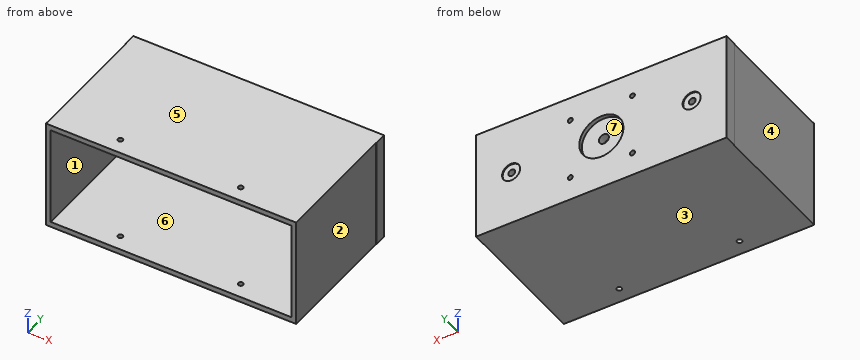
```python
from build123d import *

# Parameters (mm, degrees)
SKETCH_1_W                     = 125
SKETCH_1_H                     = 55
EXTRUDE_1_DEPTH                = 6
SKETCH_2_R                     = 11
CUT_EXTRUDE_1_DEPTH            = 2
CUT_EXTRUDE_2_REACH            = 70.4
SKETCH_3_R                     = 2.5
HOLE_WIZARD_M3_1_D             = 2.5
HOLE_WIZARD_M3_1_DEPTH         = 7.5
HOLE_WIZARD_M3_1_TIP           = 0.751075774
SKETCH_6_W                     = 124.723991502
SKETCH_6_H                     = 55
SKETCH_6_W_2                   = 120
SKETCH_6_H_2                   = 49.685135096
EXTRUDE_2_DEPTH                = 63.306419
HOLE_WIZARD_M3_2_D             = 2.5
HOLE_WIZARD_M3_2_DEPTH         = 2.657432452
HOLE_WIZARD_M3_3_D             = 2.5
HOLE_WIZARD_M3_1_2_D           = 3.4
HOLE_WIZARD_M3_1_2_DEPTH       = 5
HOLE_WIZARD_M3_1_2_CBORE_D     = 9
HOLE_WIZARD_M3_1_2_CBORE_DEPTH = 0.5
HOLE_WIZARD_M3_1_2_TIP         = 1.021463052


with BuildPart() as part:
    # 草图1 → 凸台-拉伸1 (new body)
    with BuildSketch(Plane(origin=(0, 0, 0), x_dir=(1, 0, 0), z_dir=(0, 1, 0))):
        Rectangle(SKETCH_1_W, SKETCH_1_H)
    extrude(amount=EXTRUDE_1_DEPTH)

    # 草图2 → 切除-拉伸1 (cut)
    with BuildSketch(Plane(origin=(0, 6, 0), x_dir=(1, 0, 0), z_dir=(0, 1, 0))):
        with Locations(Location((0, 0, 0), (0, 0, 270))):
            Circle(SKETCH_2_R)
    extrude(amount=-CUT_EXTRUDE_1_DEPTH, mode=Mode.SUBTRACT)

    # 草图3 → 切除-拉伸2 (cut, up to next)
    with BuildSketch(Plane(origin=(0, 4, 0), x_dir=(1, 0, 0), z_dir=(0, 1, 0)), mode=Mode.PRIVATE) as cut_extrude_2_sk1:
        with Locations(Location((0, 0, 0), (0, 0, 270))):
            Circle(SKETCH_3_R)
    cut_extrude_2_tool1 = extrude(cut_extrude_2_sk1.sketch, amount=-CUT_EXTRUDE_2_REACH, mode=Mode.PRIVATE) & part.part
    add(cut_extrude_2_tool1.solids().sort_by_distance((0, 4, 0))[0], mode=Mode.SUBTRACT)

    # Hole Wizard M3 _1
    with Locations(Plane(origin=(0, 6, 0), x_dir=(1, 0, 0), z_dir=(0, 1, 0))):
        with Locations((15.5, 15.657432452), (15.5, -15.342567548), (-15.5, -15.342567548), (-15.5, 15.657432452)):
            Hole(HOLE_WIZARD_M3_1_D / 2, depth=HOLE_WIZARD_M3_1_DEPTH)
            with Locations((0, 0, -(HOLE_WIZARD_M3_1_DEPTH + HOLE_WIZARD_M3_1_TIP / 2))):  # 118° drill point
                Cone(0, HOLE_WIZARD_M3_1_D / 2, HOLE_WIZARD_M3_1_TIP, mode=Mode.SUBTRACT)

    # 草图6 → 凸台-拉伸2 (add)
    with BuildSketch(Plane.XZ):
        Rectangle(SKETCH_6_W, SKETCH_6_H)
        Rectangle(SKETCH_6_W_2, SKETCH_6_H_2, mode=Mode.SUBTRACT)
    extrude(amount=EXTRUDE_2_DEPTH)

    # M3 螺纹孔2
    with Locations(Plane(origin=(0, 0, -27.5), x_dir=(-1, 0, 0), z_dir=(0, 0, -1))):
        with Locations((30, -55.806419172), (-30, -55.806419172)):
            Hole(HOLE_WIZARD_M3_2_D / 2, depth=HOLE_WIZARD_M3_2_DEPTH)

    # M3 螺纹孔3 (through all)
    with Locations(Plane.XY.offset(27.5)):
        with Locations((30, -55.806419172), (-30, -55.806419172)):
            Hole(HOLE_WIZARD_M3_3_D / 2)

    # Hole Wizard M3 _1 2
    with Locations(Plane(origin=(-45, 6, 0), x_dir=(0, 0, 1), z_dir=(0, 1, 0))):
        with Locations((0, 0), (0, 90)):
            CounterBoreHole(HOLE_WIZARD_M3_1_2_D / 2, HOLE_WIZARD_M3_1_2_CBORE_D / 2, HOLE_WIZARD_M3_1_2_CBORE_DEPTH, depth=HOLE_WIZARD_M3_1_2_DEPTH)
            with Locations((0, 0, -(HOLE_WIZARD_M3_1_2_DEPTH + HOLE_WIZARD_M3_1_2_TIP / 2))):  # 118° drill point
                Cone(0, HOLE_WIZARD_M3_1_2_D / 2, HOLE_WIZARD_M3_1_2_TIP, mode=Mode.SUBTRACT)


solid = part.part
```
Build history of the part. All positions in model axes, mm. Face numbers are marked on the shaded views. A direction names the side the tool comes from. Round coordinates to 2 decimals unless told otherwise and drop trailing zeros. Order: outer loops, then holes, each group sorted by start corner. A loop starts at its lowest first (then second) coordinate and runs counter-clockwise, first axis right, second up. Notation, with made-up numbers: (2.5, 30.5) - (22.5, 30.5) arc R11 cw to (22.5, 46.5) - close; hole circle Ø1 at (12.5, 70). An arc over 180 degrees is marked (long way). Use a Markdown table: item, result.
1) Saw through at D-D on z = -22. Write the cut outline in (x, y), and give its area (3 significant figures).
Recorded:
| item | result |
|---|---|
| outline | (-62.5, 0) - (-62.36, 0) - (-62.36, -63.31) - (-60, -63.31) - (-60, 0) - (60, 0) - (60, -63.31) - (62.36, -63.31) - (62.36, 0) - (62.5, 0) - (62.5, 6) - (-62.5, 6) - close |
| area | 1,050 mm² |
2) Saw through at B-B on y = -36. Write the cut outline in (x, z), and give its area (3 significant figures).
Recorded:
| item | result |
|---|---|
| outline | (-62.36, -27.5) - (62.36, -27.5) - (62.36, 27.5) - (-62.36, 27.5) - close; hole (-60, -24.84) - (60, -24.84) - (60, 24.84) - (-60, 24.84) - close |
| area | 898 mm² |
3) Saw through at A-A on x = 15.5. Write the cut outline in (y, z).
Recorded:
| item | result |
|---|---|
| outline | (-63.31, -27.5) - (6, -27.5) - (6, -16.91) - (0, -16.91) - (0, -24.84) - (-63.31, -24.84) - close; (-63.31, 24.84) - (0, 24.84) - (0, 16.59) - (6, 16.59) - (6, 27.5) - (-63.31, 27.5) - close; (0, -14.41) - (6, -14.41) - (6, 14.09) - (0, 14.09) - close |
4) Wall check: L1, parallel to X at y = 5, z = 0; L2, parallel to X at y = -3, z = -20; L3, parallel to Y at x = 30, z = -25.95. Give the ranges that are in metal, low to high.
Recorded:
| item | result |
|---|---|
| L1 | x = -62.5 to -46.7, -43.3 to -11, 11 to 43.3, 46.7 to 62.5 |
| L2 | x = -62.36 to -60, 60 to 62.36 |
| L3 | y = -63.31 to -57.06, -54.56 to 6 |
5) Saw through at C-C on x = -27. Write the cut outline in (y, z).
Recorded:
| item | result |
|---|---|
| outline | (-63.31, -27.5) - (6, -27.5) - (6, 27.5) - (-63.31, 27.5) - (-63.31, 24.84) - (0, 24.84) - (0, -24.84) - (-63.31, -24.84) - close |
6) Flat gauge pins, fed straight in: pin 1 Ø5 at (y, z) = (-19.5, -20.5) entering from -X; pin 2 Ø25 at (y, z) = (-19, -12) entering from +X; pin 3 Ø25 at (x, z) = (7, 3) entering from -Y. Where does each tip first touch, or does it go through?
Recorded:
| item | result |
|---|---|
| pin 1 | stops at x = -62.36 |
| pin 2 | stops at x = 62.36 |
| pin 3 | stops at y = 0 |
7) Pull direction X, two halves, no side cores. Call the marked faces 1, 2, 3 and 4: pulls with the +X half, pulls with the -X half, needs draft (parallel to the pull), parting line crosses it, or undercut.
Recorded:
| item | result |
|---|---|
| face 1 | undercut |
| face 2 | pulls with the +X half |
| face 3 | needs draft |
| face 4 | pulls with the -X half |
8) Tool access for the marked faces 5, 6 and 7: list every direction of +Z, -Z, +X, -X, +Y, -Y with a clear straight run to the whole face (end or side of a thin tool).
Recorded:
| item | result |
|---|---|
| face 5 | +Z, +X, -X, +Y, -Y |
| face 6 | -Y |
| face 7 | +Y |
